from build123d import *

# Parameters (mm, degrees)
SKETCH2_R               = 1.8
CUT_EXTRUDE1_DEPTH      = 10
SKETCH3_W               = 5.6
SKETCH3_H               = 10.691433847
CUT_EXTRUDE2_DEPTH      = 2.4
BOSS_EXTRUDE1_DEPTH     = 2.5
SKETCH5_R               = 1.8
CUT_EXTRUDE3_DEPTH      = 92.440311816
SKETCH6_W               = 5.6
SKETCH6_H               = 10.168713577
SKETCH6_W_2             = 10.168713577
SKETCH6_H_2             = 5.6
CUT_EXTRUDE4_DEPTH      = 2.4
CUT_EXTRUDE5_DEPTH      = 95.35095389
CUT_EXTRUDE5_DEPTH_BACK = 95.35095389
SKETCH7_W               = 158.937204397
SKETCH7_H               = 33.212886659
CHAMFER1_SIZE           = 1


with BuildPart() as part:
    # Sketch1 → Revolve1 (revolve)
    with BuildSketch(Plane(origin=(0, 0, 0), x_dir=(1, 0, 0), z_dir=(0, 1, 0))):
        Polygon((43.05, 0), (43.05, 5.5), (40.025, 5.5), (40.025, 8.05), (33.75, 8.05), (33.75, 11.55), (47.85, 11.55), (47.85, 26.05), (33.75, 26.05), (33.75, 31.05), (47.95, 31.05), (47.95, 29.05), (50.35, 29.05), (50.35, 24.05), (53.5, 24.05), (53.5, 31.05), (55, 31.05), (55, 20.475), (63, 20.475), (63, 10.475), (55, 10.475), (55, 0), align=None)
    revolve(axis=Axis((0, 0, 39.851832449), (0, 0, -1)))

    # Sketch2 → Cut-Extrude1 (cut)
    with BuildSketch(Plane.XY):
        with Locations((0, 50)):
            Circle(SKETCH2_R)
        with Locations((43.301270189, 25)):
            Circle(SKETCH2_R)
        with Locations((43.301270189, -25)):
            Circle(SKETCH2_R)
        with Locations((0, -50)):
            Circle(SKETCH2_R)
        with Locations((-43.301270189, -25)):
            Circle(SKETCH2_R)
        with Locations((-43.301270189, 25)):
            Circle(SKETCH2_R)
    extrude(amount=-CUT_EXTRUDE1_DEPTH, mode=Mode.SUBTRACT)

    # Sketch3 → Cut-Extrude2 (cut)
    with BuildSketch(Plane.XY.offset(-5)):
        with Locations((0, 52.545716924)):
            Rectangle(SKETCH3_W, SKETCH3_H)
        Polygon((51.535452373, 26.520845793), (48.735452373, 31.370588054), (39.476399059, 26.024871131), (42.276399059, 21.175128869), align=None)
        Polygon((48.735452373, -31.370588054), (51.535452373, -26.520845793), (42.276399059, -21.175128869), (39.476399059, -26.024871131), align=None)
        with Locations((0, -52.545716924)):
            Rectangle(SKETCH3_W, SKETCH3_H)
        Polygon((-51.535452373, -26.520845793), (-48.735452373, -31.370588054), (-39.476399059, -26.024871131), (-42.276399059, -21.175128869), align=None)
        Polygon((-48.735452373, 31.370588054), (-51.535452373, 26.520845793), (-42.276399059, 21.175128869), (-39.476399059, 26.024871131), align=None)
    extrude(amount=-CUT_EXTRUDE2_DEPTH, mode=Mode.SUBTRACT)

    # Sketch4 → Boss-Extrude1 (add)
    with BuildSketch(Plane.XY.offset(-5.5)):
        with BuildLine():
            Line((-2.45, 42.980228012), (-2.45, 39.949945244))
            ThreePointArc((-2.45, 39.949945244), (0, 40.025), (2.45, 39.949945244))
            Line((2.45, 39.949945244), (2.45, 42.980228012))
            ThreePointArc((2.45, 42.980228012), (0, 43.05), (-2.45, 42.980228012))
        make_face()
    extrude(amount=BOSS_EXTRUDE1_DEPTH)

    # Sketch5 → Cut-Extrude3 (cut, through all)
    with BuildSketch(Plane.XY.offset(-10.475)):
        with Locations((0, 59)):
            Circle(SKETCH5_R)
        with Locations((59, 0)):
            Circle(SKETCH5_R)
        with Locations((0, -59)):
            Circle(SKETCH5_R)
        with Locations((-59, 0)):
            Circle(SKETCH5_R)
    extrude(amount=-CUT_EXTRUDE3_DEPTH, mode=Mode.SUBTRACT)

    # Sketch6 → Cut-Extrude4 (cut)
    with BuildSketch(Plane.XY.offset(-16.775)):
        with Locations((0, 61.284356789)):
            Rectangle(SKETCH6_W, SKETCH6_H)
        with Locations((61.284356789, 0)):
            Rectangle(SKETCH6_W_2, SKETCH6_H_2)
        with Locations((0, -61.284356789)):
            Rectangle(SKETCH6_W, SKETCH6_H)
        with Locations((-61.284356789, 0)):
            Rectangle(SKETCH6_W_2, SKETCH6_H_2)
    extrude(amount=-CUT_EXTRUDE4_DEPTH, mode=Mode.SUBTRACT)

    # Sketch7 → Cut-Extrude5 (cut, two sides: drawn at the far end of the back side and taken through both)
    with BuildSketch(Plane(origin=(0, 0, 0), x_dir=(1, 0, 0), z_dir=(0, 1, 0)).offset(-CUT_EXTRUDE5_DEPTH_BACK)):
        with Locations((-3.919975894, 32.08144333)):
            Rectangle(SKETCH7_W, SKETCH7_H)
    extrude(amount=CUT_EXTRUDE5_DEPTH + CUT_EXTRUDE5_DEPTH_BACK, mode=Mode.SUBTRACT)

    # Chamfer1
    chamfer1_edges = [part.edges().sort_by_distance(p)[0] for p in [
        (-55, 0, -10.475),
    ]]
    chamfer(chamfer1_edges, length=CHAMFER1_SIZE)


solid = part.part
For this review, take the finished solid that the model builds, in its own axes (mm). A direction names the side the tool comes from. Coordinates: 2 decimals unless noted, no trailing zeros. Order: outer loops, then holes, each group sorted by start corner. A loop starts at its lowest first (then second) coordinate and runs counter-clockwise, first axis right, second up. Notation, with made-up numbers: (18, -5) -> (27, -5) arc R19 ccw to (27, 10) -> close; hole circle Ø6 at (-23, -40). An arc over 180 degrees is marked (long way). Return JSON: item names as keys, results as strings.
1. For line 1 (Y direction, x = 0, z = -2.9); line 2 (X direction, y = 1.5, z = -2); line 3 (X direction, y = 0, z = -7.3) (3 decimals), list the stretches that pass through material, from the lowest coordinate up. Write a range as from..to.
Answer block:
{"line 1": "-55..-51.8, -48.2..-43.05, 43.05..48.2, 51.8..55", "line 2": "-54.98..-43.02, 43.02..54.98", "line 3": "-55..-40.025, 40.025..55"}
2. We need section B-B on x = -59. Write out the cut boundary in (y, z) (3 decimals).
Answer block:
{"outline": "(-22.091, -15.475) -> (-1.8, -15.475) -> (-1.8, -10.475) -> (-22.091, -10.475) -> close; (1.8, -15.475) -> (22.091, -15.475) -> (22.091, -10.475) -> (1.8, -10.475) -> close"}
3. Machinability: for faces 1 (the flat face through (33, 10, -11.55)), 2 (the flat face through (45.2, -25.5, -7.4)), 3 (the cylindrical face through (-0.234, -48.215, -8.682)), 4 (the flat face through (0, -52, -7.4)), which of the approach directions +Z, -Z, +X, -X, +Y, -Y give a long, thin tool a straight path to every point of the face, cutting with its end or side? Answer none if there is none.
Answer block:
{"face 1": "-Z", "face 2": "none", "face 3": "+Z", "face 4": "-Y"}
4. For pin 1 Ø3 at (x, y) = (43.3, -25) entering from +Z; pin 2 Ø1 at (x, z) = (4, -4.5) entering from +Y; pin 3 Ø6 at (x, y) = (-22, -22.5) entering from +Z, all flat-tipped, find the tip position at first contact; note any pin that passes through.
Answer block:
{"pin 1": "z = -10", "pin 2": "y = 54.89", "pin 3": "z = -8.05"}
5. The part is to be moulded in two halves that separate along Y. For faces 5 (the flat face through (-45.3, -25.5, -7.4)), 6 (the flat face through (0, -52, -5)), say which applies: +Y half, -Y half, draft (parallel to the pull), parting line (faces both ways), or undercut.
Answer block:
{"face 5": "undercut", "face 6": "draft"}
6. We need section A-A on y = 0. State how many separate pieces and enclosed holes the cut face has, and give its area (3 significant figures).
Answer block:
{"separate pieces": "4", "enclosed holes": "0", "area": "458 mm²"}
